Print and shaded views of the part. All mm, measured from the part's lowest x, y and z. A direction names the side the tool comes from. Give positions to 0.01 mm unless a question says otherwise; leave off trailing zeros. Loops run counter-clockwise (first coordinate to the right, second up) from the corner with the lowest first, then second, coordinate; pieces in that order, holes last.
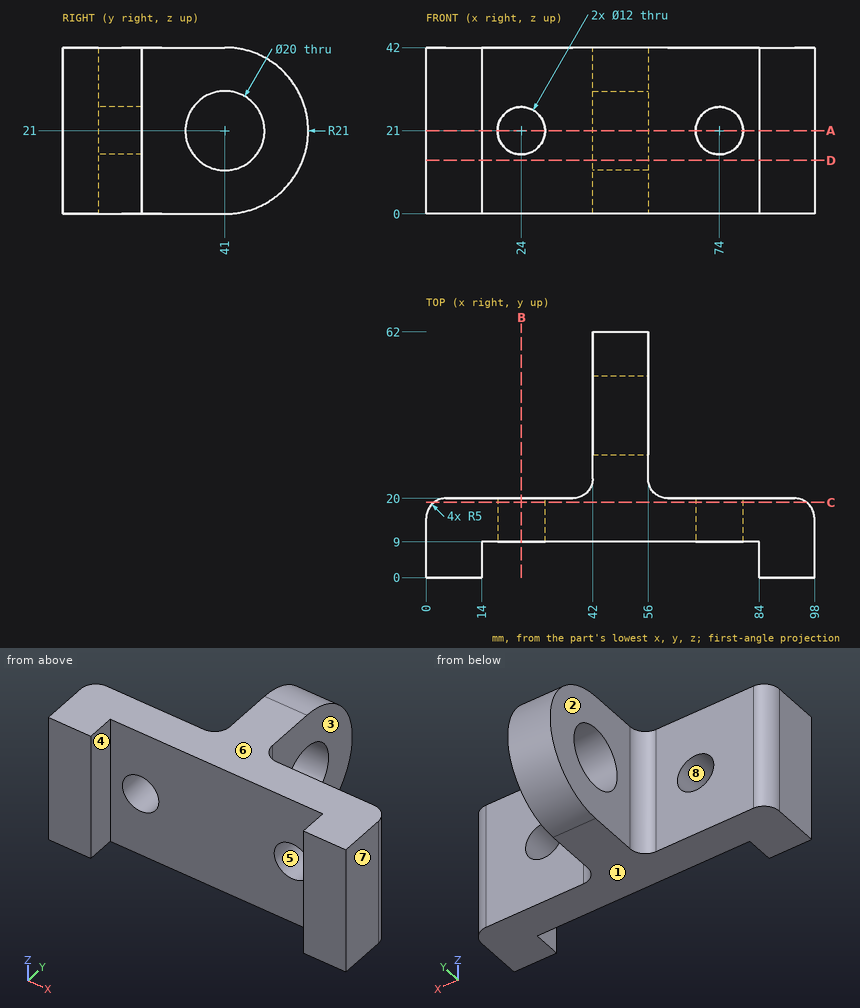
1. Drop flat-ended pins along their axis: pin 1 (23 mm diameter, centred on y = 41, z = 21, fed in from -X); pin 2 (9.5 mm diameter, centred on x = 29, z = 30.5, fed in from +Y); pin 3 (4 mm diameter, centred on y = 18, z = 20.5, fed in from +X). Give the stop position or say it passes through.
Responses:
pin 1: stops at x = 42
pin 2: stops at y = 20
pin 3: stops at x = 97.9
2. Saw through at B-B, the plane x = 24. List the corners of the cut face in (y, z).
Responses:
outline: (9, 0) - (20, 0) - (20, 15) - (9, 15) - close; (9, 27) - (20, 27) - (20, 42) - (9, 42) - close
3. Probe line 1 along X through (y, z) = (12.25, 21); line 2 along Y through (x, z) = (48, 20.5); line 3 along Z through (x, y) = (74, 11.5). List the from-to ranges inside material, lowest first.
Responses:
line 1: x = 0 to 18, 30 to 68, 80 to 98
line 2: y = 9 to 31.01, 50.99 to 61.99
line 3: z = 0 to 15, 27 to 42
4. Pull direction Z, two halves, no side cores. Call the marked faces 5, 6, 7 and 8: released by +Z, released by -Z, zero draft, split by the parting line, or undercut.
Responses:
face 5: undercut
face 6: released by +Z
face 7: zero draft
face 8: undercut
5. Saw through at A-A, the plane z = 21. List the corners of the cut face in (x, y), and give its area (3 significant figures).
Responses:
outline: (0, 0) - (14, 0) - (14, 9) - (18, 9) - (18, 20) - (5, 20) arc R5 ccw to (0, 15) - close; (30, 9) - (68, 9) - (68, 20) - (61, 20) arc R5 cw to (56, 25) - (56, 31) - (42, 31) - (42, 25) arc R5 cw to (37, 20) - (30, 20) - close; (42, 51) - (56, 51) - (56, 62) - (42, 62) - close; (80, 9) - (84, 9) - (84, 0) - (98, 0) - (98, 15) arc R5 ccw to (93, 20) - (80, 20) - close
area: 1,370 mm2
6. Tool access for the marked faces 1, 2, 3 and 4: list every direction of +Z, -Z, +X, -X, +Y, -Y with a clear straight run to the whole face (end or side of a thin tool).
Responses:
face 1: -Z, +X, -X, +Y, -Y
face 2: +Z, -Z, -X, +Y
face 3: +Z, -Z, +X, +Y
face 4: +Z, -Z, -Y
7. Saw through at D-D, the plane z = 13.5. List the corners of the cut face in (x, y).
Responses:
outline: (0, 0) - (14, 0) - (14, 9) - (84, 9) - (84, 0) - (98, 0) - (98, 15) arc R5 ccw to (93, 20) - (61, 20) arc R5 cw to (56, 25) - (56, 34.39) - (42, 34.39) - (42, 25) arc R5 cw to (37, 20) - (5, 20) arc R5 ccw to (0, 15) - close; (42, 47.61) - (56, 47.61) - (56, 60.62) - (42, 60.62) - close
8. Saw through at C-C, the plane y = 19. List the corners of the cut face in (x, z), and give its area (3 significant figures).
Responses:
outline: (2, 0) - (96, 0) - (96, 42) - (2, 42) - close; hole circle Ø12 at (24, 21); hole circle Ø12 at (74, 21)
area: 3,720 mm2
